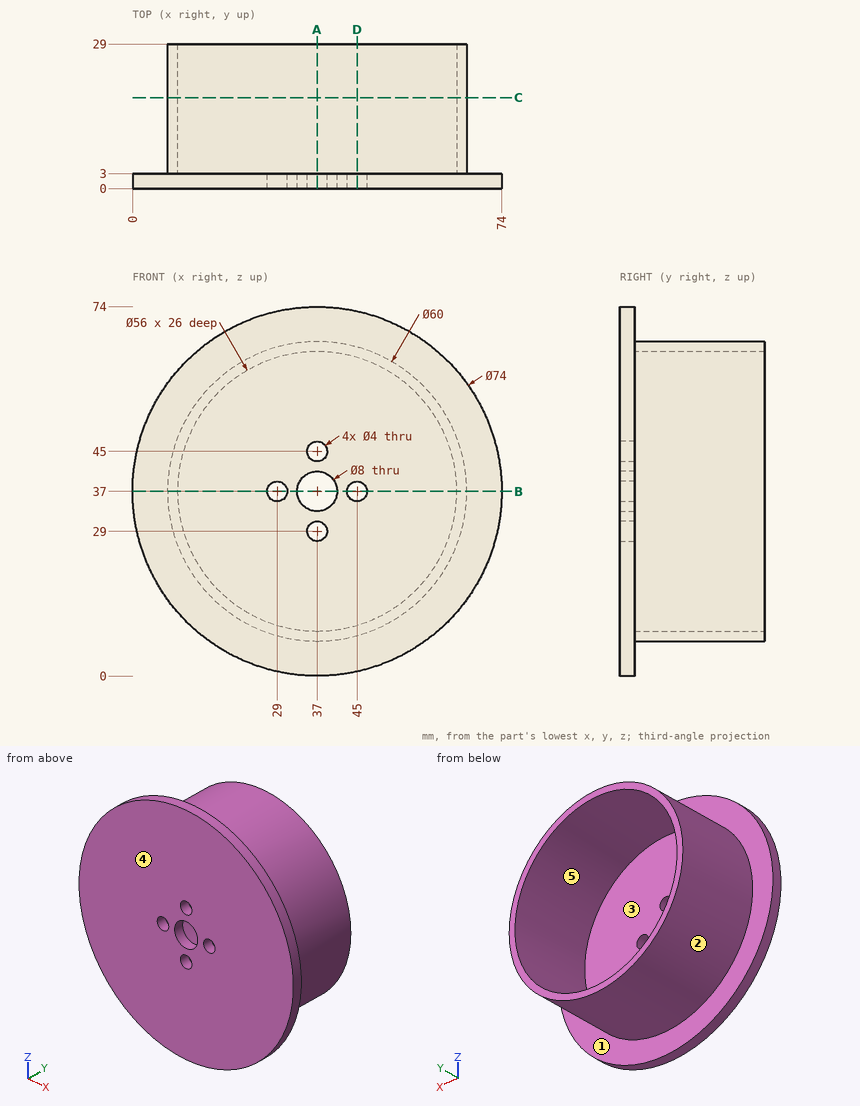
For this review, use the dimensioned drawing (mm, ordinates from the lowest corner) and the shaded views. A direction names the side the tool comes from. Give positions to 0.01 mm unless a question says otherwise; leave off trailing zeros. Order: outer loops, then holes, each group sorted by start corner. A loop starts at its lowest first (then second) coordinate and runs counter-clockwise, first axis right, second up. Notation, with made-up numbers: (28, 48.25) - (45, 48.25) arc R34 cw to (45, 81.25) - close; hole circle Ø4 at (64, 89). An arc over 180 degrees is marked (long way). Use CSV: the item, a comma, the result in double quotes. Start each with the question number.
Q1. We need section D-D, the plane x = 45. Write out the cut boundary in (y, z).
Q2. The part is to be moulded in two halves that separate along Z. For the marked faces 1, 2 and 3, say which applies: +Z half, -Z half, draft (parallel to the pull), parting line (faces both ways), or undercut.
Q3. Clearance check with flat-ended pins moving along their axes: pin 1 Ø6 at (x, y) = (51.5, 11.5) entering from -Z; pin 2 Ø10 at (y, z) = (9, 22.5) entering from -X; pin 3 Ø22 at (x, z) = (34.5, 48) entering from +Y; pin 4 Ø5 at (x, z) = (37, 37) entering from +Y. State where each tip first meets the part, or that it passes through.
Q4. To check wall thickness, follow line 1 along X through (y, z) = (2.1, 37); line 2 along Y through (x, z) = (70, 29.5); line 3 along X through (y, z) = (18.5, 37). State the ranges of each line that lie inside material, in increasing order. Write a range as [from, to].
Q5. We need section C-C, the plane y = 18.25. Write out the cut boundary in (x, z).
Q6. We need section B-B, the plane z = 37. Write out the cut boundary in (x, y), and give its area (3 significant figures).
Q7. We need section A-A, the plane x = 37. Write out the cut boundary in (y, z).
Q8. Tool access review of the marked faces 4 and 5: name each direction out of +Z, -Z, +X, -X, +Y, -Y from which nothing blocks a thin tool from reaching the whole face with its end or side.
Outcome:
1,outline,"(0, 0.88) - (3, 0.88) - (3, 8.09) - (29, 8.09) - (29, 10.17) - (3, 10.17) - (3, 35) - (0, 35) - close; (0, 39) - (3, 39) - (3, 63.83) - (29, 63.83) - (29, 65.91) - (3, 65.91) - (3, 73.12) - (0, 73.12) - close"
2,face 1,"draft"
2,face 2,"parting line"
2,face 3,"undercut"
3,pin 1,"stops at z = 9.29"
3,pin 2,"stops at x = 8.54"
3,pin 3,"stops at y = 3"
3,pin 4,"passes through"
4,line 1,"x = [0, 27], [31, 33], [41, 43], [47, 74]"
4,line 2,"y = [0, 3]"
4,line 3,"x = [7, 9], [65, 67]"
5,outline,"circle Ø60 at (37, 37); hole circle Ø56 at (37, 37)"
6,outline,"(0, 0) - (27, 0) - (27, 3) - (9, 3) - (9, 29) - (7, 29) - (7, 3) - (0, 3) - close; (31, 0) - (33, 0) - (33, 3) - (31, 3) - close; (41, 0) - (43, 0) - (43, 3) - (41, 3) - close; (47, 0) - (74, 0) - (74, 3) - (67, 3) - (67, 29) - (65, 29) - (65, 3) - (47, 3) - close"
6,area,"278 mm^2"
7,outline,"(0, 0) - (3, 0) - (3, 7) - (29, 7) - (29, 9) - (3, 9) - (3, 27) - (0, 27) - close; (0, 31) - (3, 31) - (3, 33) - (0, 33) - close; (0, 41) - (3, 41) - (3, 43) - (0, 43) - close; (0, 47) - (3, 47) - (3, 65) - (29, 65) - (29, 67) - (3, 67) - (3, 74) - (0, 74) - close"
8,face 4,"+Z, -Z, +X, -X, -Y"
8,face 5,"+Y"
